```python
from build123d import *

# Parameters (mm, degrees)
SKETCH1_R           = 2.3
SKETCH1_R_2         = 1.609204822
BOSS_EXTRUDE1_DEPTH = 3
SKETCH2_R           = 2.1
BOSS_EXTRUDE2_DEPTH = 3


with BuildPart() as part:
    # Sketch1 → Boss-Extrude1 (new body)
    with BuildSketch(Plane(origin=(0, 0, 0), x_dir=(1, 0, 0), z_dir=(0, 1, 0))):
        Polygon((-30.75, 58.5), (-30.75, 19.5), (-27.75, 19.5), (-27.75, -19.5), (-30.75, -19.5), (-30.75, -58.5), (-14, -58.5), (-14, -55.5), (14, -55.5), (14, -58.5), (30.75, -58.5), (30.75, -19.5), (27.75, -19.5), (27.75, 19.5), (30.75, 19.5), (30.75, 58.5), (14, 58.5), (14, 55.5), (-14, 55.5), (-14, 58.5), align=None)
        with Locations(Location((0, 37.5, 0), (0, 0, 270))):
            Circle(SKETCH1_R, mode=Mode.SUBTRACT)
        with Locations(Location((0, -37.5, 0), (0, 0, 270))):
            Circle(SKETCH1_R, mode=Mode.SUBTRACT)
        with Locations(Location((-22, -42.94, 0), (0, 0, 270))):
            Circle(SKETCH1_R_2, mode=Mode.SUBTRACT)
        with Locations(Location((22, -42.94, 0), (0, 0, 270))):
            Circle(SKETCH1_R_2, mode=Mode.SUBTRACT)
        with Locations(Location((22, 42.94, 0), (0, 0, 270))):
            Circle(SKETCH1_R_2, mode=Mode.SUBTRACT)
        with Locations(Location((-22, 42.94, 0), (0, 0, 270))):
            Circle(SKETCH1_R_2, mode=Mode.SUBTRACT)
    extrude(amount=BOSS_EXTRUDE1_DEPTH)

    # Sketch2 → Boss-Extrude2 (add)
    with BuildSketch(Plane(origin=(0, 3, 0), x_dir=(1, 0, 0), z_dir=(0, 1, 0))):
        Polygon((-24, 58.5), (-15, 67.5), (15, 67.5), (24, 58.5), align=None)
        with Locations(Location((0, 63, 0), (0, 0, 270))):
            Circle(SKETCH2_R, mode=Mode.SUBTRACT)
        with Locations(Location((12.7, 63, 0), (0, 0, 270))):
            Circle(SKETCH2_R, mode=Mode.SUBTRACT)
        with Locations(Location((-12.7, 63, 0), (0, 0, 270))):
            Circle(SKETCH2_R, mode=Mode.SUBTRACT)
    boss_extrude2 = extrude(amount=-BOSS_EXTRUDE2_DEPTH)

    # Mirror1: Boss-Extrude2 across plane
    add(boss_extrude2.mirror(Plane.XY))


solid = part.part
```
For this review, take the finished solid that the model builds, in its own axes (mm). A direction names the side the tool comes from. Round coordinates to 2 decimals unless told otherwise and drop trailing zeros. Write each loop counter-clockwise with the first axis right and the second up, starting at its lowest first coordinate (ties: lowest second). Pieces come first, ordered by that corner, then holes.
1) Mouldability with a two-part tool opening along Z and no side actions: class faces 4 (the face through (-19.6, 1.5, 62.9)), 5 (the face through (-13.5, 1.52, 61.06)), 6 (the face through (-30.75, 1, -39)) as +Z half, -Z half, draft (parallel to the pull), parting line (faces both ways), or undercut.
Answer below:
face 4: +Z half
face 5: undercut
face 6: draft
2) Take a section at A-A on z = -42.94. Give the boundary of the cut face in (x, y).
Answer below:
outline: (-30.75, 0) - (-23.61, 0) - (-23.61, 3) - (-30.75, 3) - close; (-20.39, 0) - (20.39, 0) - (20.39, 3) - (-20.39, 3) - close; (23.61, 0) - (30.75, 0) - (30.75, 3) - (23.61, 3) - close
3) Take a section at C-C on x = -12.7. Give the boundary of the cut face in (y, z), then the cut area to 3 significant figures.
Answer below:
outline: (0, -67.5) - (3, -67.5) - (3, -65.1) - (0, -65.1) - close; (0, -60.9) - (3, -60.9) - (3, -58.5) - (0, -58.5) - close; (0, -55.5) - (3, -55.5) - (3, 55.5) - (0, 55.5) - close; (0, 58.5) - (3, 58.5) - (3, 60.9) - (0, 60.9) - close; (0, 65.1) - (3, 65.1) - (3, 67.5) - (0, 67.5) - close
area: 362 mm2
4) Insertion check: pin 1 Ø1 at (x, y) = (-21, 0.5) entering from +Z; pin 2 Ø3 at (x, z) = (0, -37.5) entering from +Y; pin 3 Ø1.5 at (y, z) = (2, 0) entering from -X; pin 4 Ø0.9 at (x, y) = (-28, 1) entering from -Z. Each pin has a flat end and moves straight along its axis. Give the tip position at first contact, or say it passes through.
Answer below:
pin 1: stops at z = 62
pin 2: passes through
pin 3: stops at x = -27.75
pin 4: stops at z = -58.5
5) Take a section at B-B on x = 6.5. Give the boundary of the cut face in (y, z), then the cut area to 3 significant figures.
Answer below:
outline: (0, -67.5) - (3, -67.5) - (3, -58.5) - (0, -58.5) - close; (0, -55.5) - (3, -55.5) - (3, 55.5) - (0, 55.5) - close; (0, 58.5) - (3, 58.5) - (3, 67.5) - (0, 67.5) - close
area: 387 mm2
6) Machinability: for faces 1 (the face through (0, 1, 55.5)), 2 (the face through (29, 1, -19.5)), 3 (the face through (-29, 1, 19.5)), which of the approach directions +Z, -Z, +X, -X, +Y, -Y give a long, thin tool a straight path to every point of the face, cutting with its end or side? Answer none if there is none.
Answer below:
face 1: +Y, -Y
face 2: +X, +Y, -Y
face 3: -X, +Y, -Y
7) Take a section at D-D on z = 63. Give the boundary of the cut face in (x, y).
Answer below:
outline: (-19.5, 0) - (-14.8, 0) - (-14.8, 3) - (-19.5, 3) - close; (-10.6, 0) - (-2.1, 0) - (-2.1, 3) - (-10.6, 3) - close; (2.1, 0) - (10.6, 0) - (10.6, 3) - (2.1, 3) - close; (14.8, 0) - (19.5, 0) - (19.5, 3) - (14.8, 3) - close
8) For line 1 along X through (y, z) = (2.3, 63); line 2 along Z through (x, y) = (5, 2.45); line 3 along X through (y, z) = (1.1, -42.94), list the stretches that pass through material, from the lowest coordinate up.
Answer below:
line 1: x = -19.5 to -14.8, -10.6 to -2.1, 2.1 to 10.6, 14.8 to 19.5
line 2: z = -67.5 to -58.5, -55.5 to 55.5, 58.5 to 67.5
line 3: x = -30.75 to -23.61, -20.39 to 20.39, 23.61 to 30.75
